```python
from build123d import *

# Parameters (mm, degrees)
F1_DEPTH = 19.05
F2_R     = 3.175
F3_DEPTH = 12.7


with BuildPart() as f1:
    # F0 (on Right) → F1 (new body, symmetric)
    with BuildSketch(Plane.YZ):
        with BuildLine():
            Line((19.05, 0), (12.7, 0))
            ThreePointArc((12.7, 0), (0, -12.7), (-12.7, 0))
            Line((-12.7, 0), (-19.05, 0))
            ThreePointArc((-19.05, 0), (0, -19.05), (19.05, 0))
        make_face()
        with BuildLine():
            ThreePointArc((-12.7, 0), (0, 12.7), (12.7, 0))
            Line((12.7, 0), (19.05, 0))
            ThreePointArc((19.05, 0), (0, 19.05), (-19.05, 0))
            Line((-19.05, 0), (-12.7, 0))
        make_face()
        with BuildLine():
            Line((19.05, -25.4), (19.05, 0))
            ThreePointArc((19.05, 0), (0, -19.05), (-19.05, 0))
            Line((-19.05, 0), (-19.05, -25.4))
            Line((-19.05, -25.4), (19.05, -25.4))
        make_face()
    extrude(amount=F1_DEPTH, both=True)

    # F2 (on face) → F3 (cut)
    with BuildSketch(Plane(origin=(0, 0, -25.4), x_dir=(1, 0, 0), z_dir=(0, 0, -1))):
        with Locations((0, 14.2748)):
            Circle(F2_R)
        with Locations((0, -14.2748)):
            Circle(F2_R)
    extrude(amount=-F3_DEPTH, mode=Mode.SUBTRACT)


solid = f1.part
```
CAD build for the part. Positions are in the model's coordinates, mm. A direction names the side the tool comes from. Give positions to 0.01 mm unless a question says otherwise; leave off trailing zeros. Order: outer loops, then holes, each group sorted by start corner. A loop starts at its lowest first (then second) coordinate and runs counter-clockwise, first axis right, second up.
(1) Tool access for faces 4 (the flat face through (0, -14, -12.7)), 5 (the flat face through (19.05, 0, -13)): list every direction of +Z, -Z, +X, -X, +Y, -Y with a clear straight run to the whole face (end or side of a thin tool).
(2) Saw through at C-C, the plane z = 11. Give the cut face in (x, y), then the cut area to 3 significant figures.
(3) Saw through at D-D, the plane x = 10.5. Give the cut face in (y, z), then the cut area to 3 significant figures.
(4) Saw through at B-B, the plane x = 0. Give the cut face in (y, z), then the cut area to 3 significant figures.
(5) Saw through at A-A, the plane y = 0. Give the cut face in (x, z), then the cut area to 3 significant figures.
(6) Drill centre lines: L1, parallel to Y at x = 0, z = -22.5; L2, parallel to Z at x = 1, y = 0; L3, parallel to Y at x = -7, z = 0.5. Where is each one in solid material? Low to high.
(7) Mould opens along Y. For faces 1 (the cylindrical face through (0.267, 0.419, 19.045)), 2 (the cylindrical face through (-0.413, 11.127, -19.139)), 3 (the flat face through (0, 0, -25.4)) say: released by +Y, released by -Y, zero draft, split by the parting line, or undercut.
(8) Flat gauge pins, fed straight in: pin 1 (8 mm diameter, centred on x = -4, z = 4, fed in from -Y); pin 2 (4 mm diameter, centred on x = 10.5, z = 4.5, fed in from -Y); pin 3 (5 mm diameter, centred on x = 0, y = -14.27, fed in from +Z); pin 4 (10 mm diameter, centred on x = -3.5, z = 11, fed in from +Y). Where does each tip first touch, or does it go through?
Results found:
1. face 4: -Z
1. face 5: +Z, -Z, +X, +Y, -Y
2. outline: (-19.05, -15.55) - (19.05, -15.55) - (19.05, -6.35) - (-19.05, -6.35) - close; (-19.05, 6.35) - (19.05, 6.35) - (19.05, 15.55) - (-19.05, 15.55) - close
2. area: 701 mm2
3. outline: (-19.05, -25.4) - (19.05, -25.4) - (19.05, 0) arc R19.05 ccw to (-19.05, 0) - close; hole circle Ø25.4 at (0, 0)
3. area: 1,030 mm2
4. outline: (-19.05, -25.4) - (-17.45, -25.4) - (-17.45, -12.7) - (-11.1, -12.7) - (-11.1, -25.4) - (11.1, -25.4) - (11.1, -12.7) - (17.45, -12.7) - (17.45, -25.4) - (19.05, -25.4) - (19.05, 0) arc R19.05 ccw to (-19.05, 0) - close; hole circle Ø25.4 at (0, 0)
4. area: 870 mm2
5. outline: (-19.05, -25.4) - (19.05, -25.4) - (19.05, -12.7) - (-19.05, -12.7) - close; (-19.05, 12.7) - (19.05, 12.7) - (19.05, 19.05) - (-19.05, 19.05) - close
5. area: 726 mm2
6. L1: y = -19.05 to -17.45, -11.1 to 11.1, 17.45 to 19.05
6. L2: z = -25.4 to -12.7, 12.7 to 19.05
6. L3: y = -19.04 to -12.69, 12.69 to 19.04
7. face 1: split by the parting line
7. face 2: undercut
7. face 3: zero draft
8. pin 1: stops at y = -19.05
8. pin 2: stops at y = -18.89
8. pin 3: stops at z = 14.98
8. pin 4: stops at y = 18.08
